Here's how the part is built. I have some questions about the finished solid (model axes, mm). Give positions to 0.01 mm unless a question says otherwise; leave off trailing zeros. Loops run counter-clockwise (first coordinate to the right, second up) from the corner with the lowest first, then second, coordinate; pieces in that order, holes last. Notation, with made-up numbers: (-36.5, -36.5) - (-13.5, -36.5) arc R23 cw to (-13.5, -12.5) - close; hole circle Ø11 at (58.25, 24.5). An arc over 180 degrees is marked (long way). Put each result on its own line as item: value. Start each with the question number.
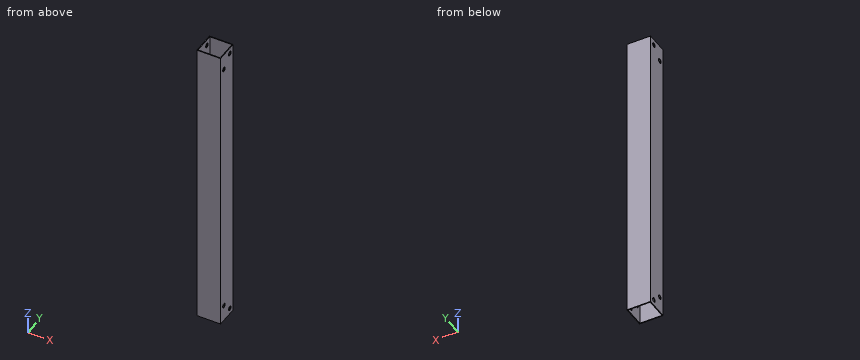
from build123d import *

# Parameters (mm, degrees)
ESQUISSE1_W             = 15.90910635
ESQUISSE1_H             = 15
ESQUISSE1_W_2           = 14.84849926
ESQUISSE1_H_2           = 14
BOSS_EXTRU_1_DEPTH      = 200
ESQUISSE6_R             = 1.5
ENL_V_MAT_EXTRU_7_DEPTH = 20


with BuildPart() as part:
    # Esquisse1 → Boss.-Extru.1 (new body)
    with BuildSketch(Plane.XY):
        with Locations((7.954553175, 7.5)):
            Rectangle(ESQUISSE1_W, ESQUISSE1_H)
        with Locations((7.954553175, 7.5)):
            Rectangle(ESQUISSE1_W_2, ESQUISSE1_H_2, mode=Mode.SUBTRACT)
    extrude(amount=-BOSS_EXTRU_1_DEPTH)

    # Esquisse6 → Enlèv. mat.-Extru.7 (cut)
    with BuildSketch(Plane(origin=(15.90910635, 0, 0), x_dir=(0, 0, -1), z_dir=(1, 0, 0))):
        with Locations(Location((4, 11, 0), (0, 0, 180))):
            Circle(ESQUISSE6_R)
        with Locations(Location((11, 4, 0), (0, 0, 180))):
            Circle(ESQUISSE6_R)
        with Locations(Location((189, 4, 0), (0, 0, 180))):
            Circle(ESQUISSE6_R)
        with Locations(Location((196, 11, 0), (0, 0, 180))):
            Circle(ESQUISSE6_R)
    extrude(amount=-ENL_V_MAT_EXTRU_7_DEPTH, mode=Mode.SUBTRACT)


solid = part.part
1) Suppose I cut it at B-B on z = -149.5. Please give me the cut outline in (x, y).
2) Suppose I cut it at C-C on y = 7.5. Please give me the cut outline in (x, z).
3) I'm going to push a flat-ended pin straight in: P1, Ø1, axis at x = 4.5, y = 2.5, coming from the +Z side. Where does the tip first touch, or does it pass through?
4) Suppose I cut it at A-A on x = 2.25. Please give me the cut outline in (y, z).
5) I need wall thicknesses on line 1 (Z direction, x = 15.7, y = 11); line 2 (Z direction, x = 15.6, y = 4); line 3 (Y direction, x = 15.7, z = -4). Which ranges of each line are inside material? Lowest first, please.
Ans:
1. outline: (0, 0) - (15.91, 0) - (15.91, 15) - (0, 15) - close; hole (0.53, 0.5) - (15.38, 0.5) - (15.38, 14.5) - (0.53, 14.5) - close
2. outline: (0, -200) - (0.53, -200) - (0.53, 0) - (0, 0) - close; (15.38, -200) - (15.91, -200) - (15.91, 0) - (15.38, 0) - close
3. P1: passes through
4. outline: (0, -200) - (0.5, -200) - (0.5, 0) - (0, 0) - close; (14.5, -200) - (15, -200) - (15, 0) - (14.5, 0) - close
5. line 1: z = -200 to -197.5, -194.5 to -5.5, -2.5 to 0
5. line 2: z = -200 to -190.5, -187.5 to -12.5, -9.5 to 0
5. line 3: y = 0 to 9.5, 12.5 to 15
